Part model, mm, in its own coordinate system. A direction names the side the tool comes from. Round coordinates to 2 decimals unless told otherwise and drop trailing zeros. Write each loop counter-clockwise with the first axis right and the second up, starting at its lowest first coordinate (ties: lowest second). Pieces come first, ordered by that corner, then holes. Notation, with made-up numbers: M -40,78.25 L -23,78.25 A16 ccw -23,84.25 Z; hole C -3.75,67.25 d9. An arc over 180 degrees is marked long. One line per question, with ' | ' between items. Start each with the question number.
1) Saw through at B-B (x = 0). List the corners of the cut face in (y, z), plus the area to 3 significant figures.
2) Saw through at C-C (z = -10.25). List the corners of the cut face in (x, y), plus the area to 3 significant figures.
3) Mould opens along Z. For faces 5 (the face through (0, 40.996, 0)), 6 (the face through (0, 36, 9.604)), 7 (the face through (-9.726, 30.159, -7.457)), 8 (the face through (0, 36, -9.604)) say: pulls with the +Z half, pulls with the -Z half, needs draft (parallel to the pull), parting line crosses it, or undercut.
4) Saw through at D-D (y = 22). List the corners of the cut face in (x, z).
5) Wall check: probe 1 along Z at (x, y) = (0, 31); probe 2 along Y at (x, z) = (5.25, -5.25); probe 3 along Z at (x, y) = (2.25, 37). Give the ranges that are in metal, low to high. Write a range as [from, to].
6) Tool access for faces 1 (the face through (-9, 31.725, 4)), 2 (the face through (8.354, 36.348, 4.737)), 3 (the face through (-5, 28.55, -5)), 4 (the face through (8.28, 36.348, -4.866)): list every direction of +Z, -Z, +X, -X, +Y, -Y with a clear straight run to the whole face (end or side of a thin tool).
7) Saw through at A-A (y = 33.5). List the corners of the cut face in (x, z), plus the area to 3 significant figures.
8) Drop flat-ended pins along their axis: pin 1 Ø6 at (x, z) = (0, 3.5) entering from -Y; pin 2 Ø10 at (x, y) = (-4.5, 23) entering from -Z; pin 3 Ø4 at (y, z) = (8.5, -3.5) entering from -X; pin 4 Ø3 at (x, y) = (-7, 11.5) entering from +Z. Give the stop position or say it passes through.
```python
from build123d import *

# Parameters (mm, degrees)
SKETCH2_W          = 10.668
SKETCH2_H          = 4.111930553
CUT_EXTRUDE1_DEPTH = 9.271
CIRPATTERN1_COUNT  = 6
CHAMFER1_SIZE      = 1.16332


with BuildPart() as part:
    # Sketch1 → Revolve1 (revolve)
    with BuildSketch(Plane.XY):
        Polygon((0, 0), (6.35, 0), (6.35, 28.5496), (12.2555, 28.5496), (12.2555, 31.7246), (10.9855, 31.7246), (10.9855, 40.9956), (0, 40.9956), align=None)
    revolve(axis=Axis((0, 40.9956, 0), (0, -1, 0)))

    # Sketch2 → Cut-Extrude1 (cut)
    with BuildSketch(Plane(origin=(0, 40.9956, 0), x_dir=(1, 0, 0), z_dir=(0, 1, 0))):
        with Locations((0, 11.659592417)):
            Rectangle(SKETCH2_W, SKETCH2_H)
    cut_extrude1 = extrude(amount=-CUT_EXTRUDE1_DEPTH, mode=Mode.SUBTRACT)

    # CirPattern1: Cut-Extrude1 ×6 about axis
    cirpattern1_axis = Axis((0, 0, 0), (0, 1, 0))
    for i in range(1, CIRPATTERN1_COUNT):
        add(cut_extrude1.rotate(cirpattern1_axis, i * 360 / CIRPATTERN1_COUNT), mode=Mode.SUBTRACT)

    # Sketch4 → Cut-Revolve1 (revolve, cut)
    with BuildSketch(Plane.XY):
        with BuildLine():
            Line((11.176, 39.4716), (11.176, 40.9956))
            Line((11.176, 40.9956), (8.6995, 40.9956))
            ThreePointArc((8.6995, 40.9956), (10.153428149, 40.584076992), (11.176, 39.4716))
        make_face()
    revolve(axis=Axis((0, -5.042553629, 0), (0, 1, 0)), mode=Mode.SUBTRACT)

    # Chamfer1
    chamfer1_edges = [part.edges().sort_by_distance(p)[0] for p in [
        (-6.35, 0, 0),
    ]]
    chamfer(chamfer1_edges, length=CHAMFER1_SIZE)


solid = part.part
```
Answer key:
1) outline: M 0,-5.19 L 1.16,-6.35 L 28.55,-6.35 L 28.55,-12.26 L 31.72,-12.26 L 31.72,-9.6 L 40.84,-9.6 A2.77 ccw 41,-8.7 L 41,8.7 A2.77 ccw 40.84,9.6 L 31.72,9.6 L 31.72,12.26 L 28.55,12.26 L 28.55,6.35 L 1.16,6.35 L 0,5.19 Z | area: 617 mm2
2) outline: M -6.72,28.55 L 6.72,28.55 L 6.72,31.72 L -6.72,31.72 Z | area: 42.7 mm2
3) face 5: needs draft | face 6: pulls with the +Z half | face 7: parting line crosses it | face 8: pulls with the -Z half
4) outline: C 0,0 d12.7
5) probe 1: z = [-12.26, 12.26] | probe 2: y = [28.55, 41] | probe 3: z = [-9.6, 9.6]
6) face 1: +Y | face 2: +Z, +X, +Y | face 3: -Y | face 4: -Z, +X, +Y
7) outline: M -10.98,-0.18 L -5.65,-9.42 A10.99 ccw -5.33,-9.6 L 5.33,-9.6 A10.99 ccw 5.65,-9.42 L 10.98,-0.18 A10.99 ccw 10.98,0.18 L 5.65,9.42 A10.99 ccw 5.33,9.6 L -5.33,9.6 A10.99 ccw -5.65,9.42 L -10.98,0.18 A10.99 ccw Z | area: 319 mm2
8) pin 1: stops at y = 0 | pin 2: stops at z = -6.35 | pin 3: stops at x = -6.17 | pin 4: stops at z = 3.17
